Input: dimensioned drawing with shaded views. Units: mm. Origin: part minimum x, y, z. Give positions to 0.01 mm unless a question says otherwise; leave off trailing zeros. Loops run counter-clockwise (first coordinate to the right, second up) from the corner with the lowest first, then second, coordinate; pieces in that order, holes last. Notation, with made-up numbers: (-6.5, 0.25) -> (27.5, 0.25) arc R22 cw to (27.5, 23.25) -> close; hole circle Ø3 at (71, -38.75). An arc over 180 degrees is marked (long way). Answer as a JSON object with one key per item and string values.
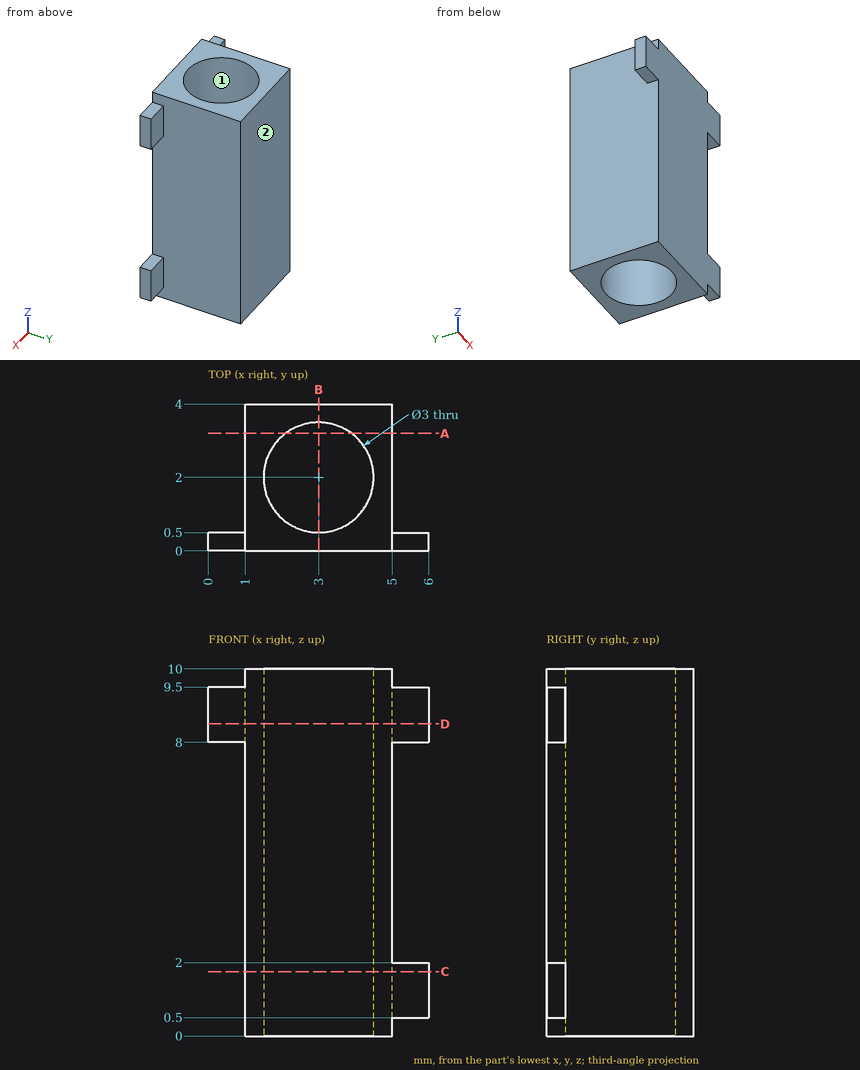
Q1. Ray query, line 1 along Y through (x, z) = (3, 5.5); line 2 along X through (y, z) = (2.1, 2.5); line 3 along Y through (x, z) = (3.95, 2.5). Return the intervals inside material, ascending.
Evaluation:
{"line 1": "y = 0 to 0.5, 3.5 to 4", "line 2": "x = 1 to 1.5, 4.5 to 5", "line 3": "y = 0 to 0.84, 3.16 to 4"}
Q2. Draft query along X for the marked faces 1 and 2. Return one class per face: +X half, -X half, draft (parallel to the pull), parting line (faces both ways), or undercut.
Evaluation:
{"face 1": "undercut", "face 2": "draft"}
Q3. Section A-A, the plane y = 3.2. Return the cut outline in (x, z), then the cut area to 3 significant figures.
Evaluation:
{"outline": "(1, 0) -> (2.1, 0) -> (2.1, 10) -> (1, 10) -> close; (3.9, 0) -> (5, 0) -> (5, 10) -> (3.9, 10) -> close", "area": "22.0 mm2"}
Q4. Pin query (flat end, axial travel): pin 1 (2 mm diameter, centred on x = 4, y = 2, fed in from +Z); pin 2 (0.8 mm diameter, centred on x = 5.5, z = 1, fed in from +Y); pin 3 (1.2 mm diameter, centred on y = 1.5, z = 5.5, fed in from -X); pin 4 (0.6 mm diameter, centred on x = 5.5, y = 0, fed in from +Z). Return the tip coordinate at first contact, or that it passes through.
Evaluation:
{"pin 1": "stops at z = 10", "pin 2": "stops at y = 0.5", "pin 3": "stops at x = 1", "pin 4": "stops at z = 9.5"}
Q5. Section B-B, the plane x = 3. Return the cut outline in (y, z).
Evaluation:
{"outline": "(0, 0) -> (0.5, 0) -> (0.5, 10) -> (0, 10) -> close; (3.5, 0) -> (4, 0) -> (4, 10) -> (3.5, 10) -> close"}
Q6. Section C-C, the plane z = 1.75. Return the cut outline in (x, y), then the cut area to 3 significant figures.
Evaluation:
{"outline": "(1, 0) -> (6, 0) -> (6, 0.5) -> (5, 0.5) -> (5, 4) -> (1, 4) -> close; hole circle Ø3 at (3, 2)", "area": "9.43 mm2"}
Q7. Section D-D, the plane z = 8.5. Return the cut outline in (x, y), then the cut area to 3 significant figures.
Evaluation:
{"outline": "(0, 0) -> (6, 0) -> (6, 0.5) -> (5, 0.5) -> (5, 4) -> (1, 4) -> (1, 0.5) -> (0, 0.5) -> close; hole circle Ø3 at (3, 2)", "area": "9.93 mm2"}
